Could you check a few things on this drawing? It's one solid part, dimensions in mm from its lowest x, y, z. A direction names the side the tool comes from. Coordinates: 2 decimals unless noted, no trailing zeros. Order: outer loops, then holes, each group sorted by start corner. A loop starts at its lowest first (then second) coordinate and runs counter-clockwise, first axis right, second up. Notation, with made-up numbers: M 14,-33.5 L 23,-33.5 A8 cw 23,-25.5 Z; hole C -32.75,66.25 d6. An arc over 180 degrees is marked long. Answer as CSV lines item,"result". Start each with the question number.
1. Will these pins go through, and if not, where does the flat tip stop? pin 1 (6 mm diameter, centred on x = 17.5, y = 16, fed in from +Z); pin 2 (6 mm diameter, centred on x = 21, z = 5, fed in from -Y); pin 3 (3.5 mm diameter, centred on x = 23, z = 9.5, fed in from -Y); pin 4 (3.5 mm diameter, centred on x = 23, z = 10.5, fed in from +Y).
2. If we section it at B-B (x = 13.5): List the corners of the cut face in (y, z) for me, plus the area to 3 significant figures.
3. If we mould it in two halves opening along Y, with no side actions, what happens to the marked faces 4, 5 and 6? For each: released by +Y, released by -Y, zero draft, split by the parting line, or undercut.
4. If we section it at D-D (z = 1.75): List the corners of the cut face in (x, y) for me, plus the area to 3 significant figures.
5. If we section it at A-A (y = 13.5): List the corners of the cut face in (x, z) for me, plus the area to 3 significant figures.
6. On a 3-axis mill with a long thin cutter (end or side, diameter ignored), from which of +Z, -Z, +X, -X, +Y, -Y can I reach the whole of each face in a straight line? I mean the marked faces 1, 2 and 3. Say none if no direction works.
7. If we section it at C-C (z = 5.5): List the corners of the cut face in (x, y) for me, plus the area to 3 significant figures.
8. I need wall thicknesses on line 1 along Y through (x, z) = (13.5, 6.75); line 2 along Y through (x, z) = (13.5, 2.5); line 3 along Z through (x, y) = (15.25, 25.75). Which ranges of each line are inside material? Lowest first, please. Write a range as from..to.
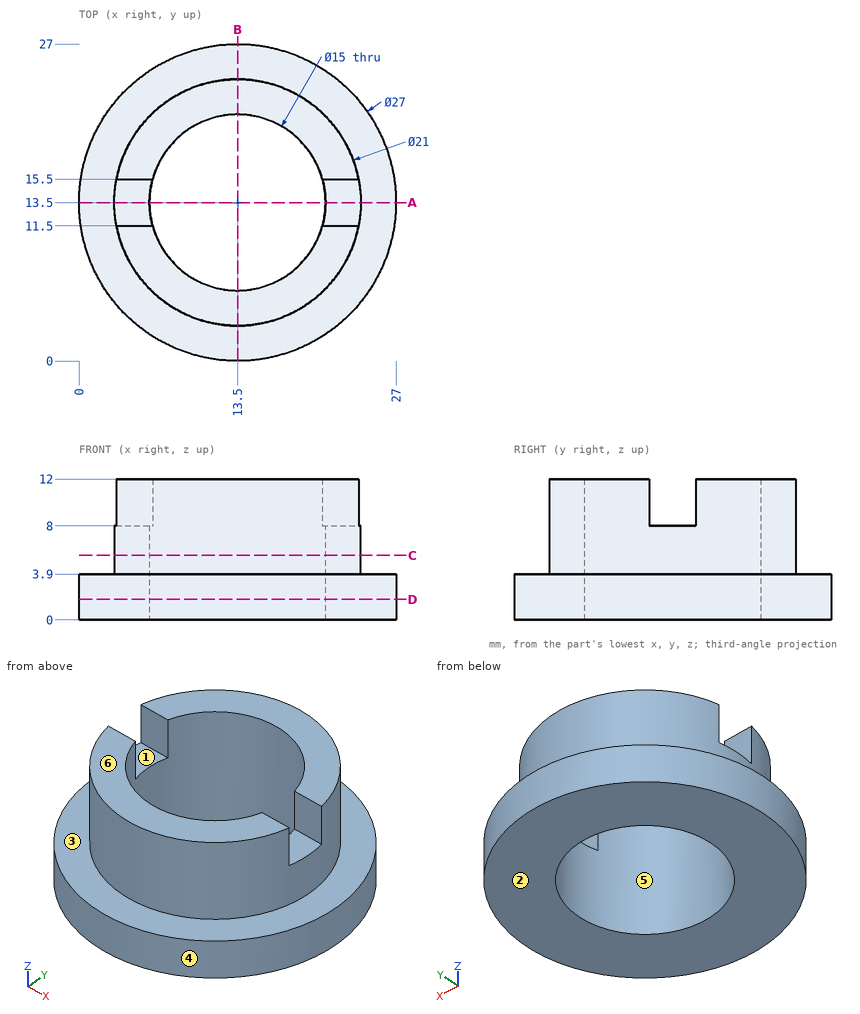
Solved:
1,pin 1,"z = 12"
1,pin 2,"y = 0.85"
1,pin 3,"y = 6.42"
1,pin 4,"y = 20.58"
2,outline,"M 0,0 L 6,0 L 6,12 L 3,12 L 3,3.9 L 0,3.9 Z; M 21,0 L 27,0 L 27,3.9 L 24,3.9 L 24,12 L 21,12 Z"
2,area,"95.4 mm²"
3,face 4,"split by the parting line"
3,face 5,"undercut"
3,face 6,"zero draft"
4,outline,"C 13.5,13.5 d27; hole C 13.5,13.5 d15"
4,area,"396 mm²"
5,outline,"M 0,0 L 6,0 L 6,8 L 3,8 L 3,3.9 L 0,3.9 Z; M 21,0 L 27,0 L 27,3.9 L 24,3.9 L 24,8 L 21,8 Z"
5,area,"71.4 mm²"
6,face 1,"+Z, +X, -X"
6,face 2,"-Z, +X, -X, +Y, -Y"
6,face 3,"+Z"
7,outline,"C 13.5,13.5 d21; hole C 13.5,13.5 d15"
7,area,"170 mm²"
8,line 1,"3..6, 21..24"
8,line 2,"0..6, 21..27"
8,line 3,"0..3.9"
